from build123d import *

# Parameters (mm, degrees)
SKETCH1_W           = 100
SKETCH1_H           = 1219.2
BOSS_EXTRUDE1_DEPTH = 13
SKETCH6_R           = 3
CUT_EXTRUDE4_DEPTH  = 20
CUT_EXTRUDE5_DEPTH  = 30


with BuildPart() as part:
    # Sketch1 → Boss-Extrude1 (new body)
    with BuildSketch(Plane(origin=(0, 0, 0), x_dir=(1, 0, 0), z_dir=(0, 1, 0))):
        Rectangle(SKETCH1_W, SKETCH1_H)
    extrude(amount=BOSS_EXTRUDE1_DEPTH)

    # Sketch6 → Cut-Extrude4 (cut)
    with BuildSketch(Plane(origin=(0, 13, 0), x_dir=(1, 0, 0), z_dir=(0, 1, 0))):
        with Locations((35, 0)):
            Circle(SKETCH6_R)
        with Locations((-35, 0)):
            Circle(SKETCH6_R)
        with Locations((35, -297.3)):
            Circle(SKETCH6_R)
        with Locations((-35, -297.3)):
            Circle(SKETCH6_R)
        with Locations((35, 600.1)):
            Circle(SKETCH6_R)
        with Locations((-35, 600.1)):
            Circle(SKETCH6_R)
        with Locations((-35, 297.3)):
            Circle(SKETCH6_R)
        with Locations((35, 297.3)):
            Circle(SKETCH6_R)
        with Locations((-35, -600.1)):
            Circle(SKETCH6_R)
        with Locations((35, -600.1)):
            Circle(SKETCH6_R)
    extrude(amount=-CUT_EXTRUDE4_DEPTH, mode=Mode.SUBTRACT)

    # Sketch7 → Cut-Extrude5 (cut)
    with BuildSketch(Plane(origin=(0, 13, 0), x_dir=(1, 0, 0), z_dir=(0, 1, 0))):
        with BuildLine():
            Line((1.3, -460.95), (1.3, -579.6))
            ThreePointArc((1.3, -579.6), (0, -580.9), (-1.3, -579.6))
            Line((-1.3, -579.6), (-1.3, -460.95))
            ThreePointArc((-1.3, -460.95), (0, -459.65), (1.3, -460.95))
        make_face()
        with BuildLine():
            Line((1.3, -312.3), (1.3, -430.95))
            ThreePointArc((1.3, -430.95), (0, -432.25), (-1.3, -430.95))
            Line((-1.3, -430.95), (-1.3, -312.3))
            ThreePointArc((-1.3, -312.3), (0, -311), (1.3, -312.3))
        make_face()
        with BuildLine():
            Line((1.3, -163.65), (1.3, -282.3))
            ThreePointArc((1.3, -282.3), (0, -283.6), (-1.3, -282.3))
            Line((-1.3, -282.3), (-1.3, -163.65))
            ThreePointArc((-1.3, -163.65), (0, -162.35), (1.3, -163.65))
        make_face()
        with BuildLine():
            Line((1.3, -15), (1.3, -133.65))
            ThreePointArc((1.3, -133.65), (0, -134.95), (-1.3, -133.65))
            Line((-1.3, -133.65), (-1.3, -15))
            ThreePointArc((-1.3, -15), (0, -13.7), (1.3, -15))
        make_face()
        with BuildLine():
            Line((1.3, 133.65), (1.3, 15))
            ThreePointArc((1.3, 15), (0, 13.7), (-1.3, 15))
            Line((-1.3, 15), (-1.3, 133.65))
            ThreePointArc((-1.3, 133.65), (0, 134.95), (1.3, 133.65))
        make_face()
        with BuildLine():
            Line((1.3, 282.3), (1.3, 163.65))
            ThreePointArc((1.3, 163.65), (0, 162.35), (-1.3, 163.65))
            Line((-1.3, 163.65), (-1.3, 282.3))
            ThreePointArc((-1.3, 282.3), (0, 283.6), (1.3, 282.3))
        make_face()
        with BuildLine():
            Line((1.3, 430.95), (1.3, 312.3))
            ThreePointArc((1.3, 312.3), (0, 311), (-1.3, 312.3))
            Line((-1.3, 312.3), (-1.3, 430.95))
            ThreePointArc((-1.3, 430.95), (0, 432.25), (1.3, 430.95))
        make_face()
        with BuildLine():
            Line((1.3, 579.6), (1.3, 460.95))
            ThreePointArc((1.3, 460.95), (0, 459.65), (-1.3, 460.95))
            Line((-1.3, 460.95), (-1.3, 579.6))
            ThreePointArc((-1.3, 579.6), (0, 580.9), (1.3, 579.6))
        make_face()
    extrude(amount=-CUT_EXTRUDE5_DEPTH, mode=Mode.SUBTRACT)


solid = part.part
Input: part model. Units: mm. Frame: model coordinates. Give positions to 0.01 mm unless a question says otherwise; leave off trailing zeros. Order: outer loops, then holes, each group sorted by start corner. A loop starts at its lowest first (then second) coordinate and runs counter-clockwise, first axis right, second up.
Q1. Section A-A on z = -245.5. Output: boundary loops of the cut face in (x, y), and give its area (3 significant figures).
Checked values:
outline: (-50, 0) - (-1.3, 0) - (-1.3, 13) - (-50, 13) - close; (1.3, 0) - (50, 0) - (50, 13) - (1.3, 13) - close
area: 1,270 mm2
Q2. Ray query, probe 1 along Z at (x, y) = (-35, 5.75); probe 2 along X at (y, z) = (5.25, -297.3); probe 3 along X at (y, z) = (6.25, 17.5). Return the intervals inside material, ascending.
Checked values:
probe 1: z = -609.6 to -603.1, -597.1 to -300.3, -294.3 to -3, 3 to 294.3, 300.3 to 597.1, 603.1 to 609.6
probe 2: x = -50 to -38, -32 to 32, 38 to 50
probe 3: x = -50 to -1.3, 1.3 to 50
Q3. Section B-B on y = 8. State how many separate pieces and enclosed holes the cut face has, and give its area (3 significant figures).
Checked values:
separate pieces: 1
enclosed holes: 18
area: 119,000 mm2
